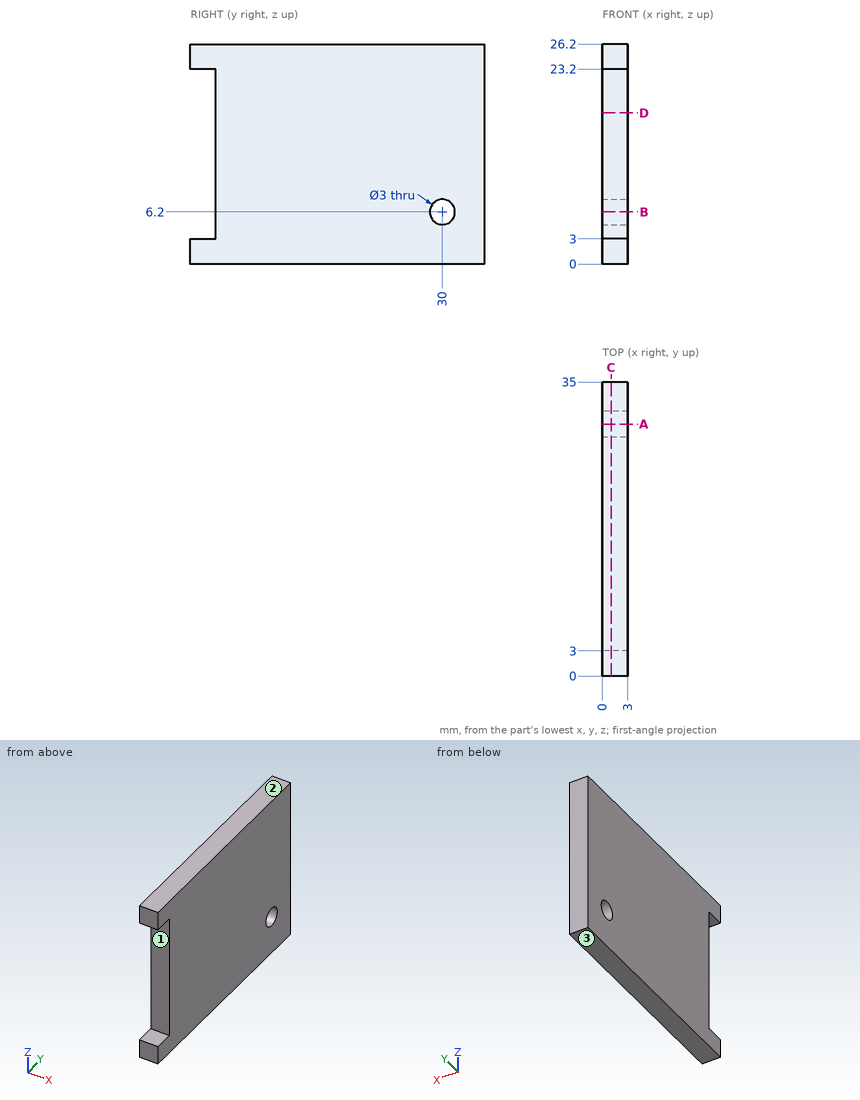
Can you work these out from the drawing? Everything is in mm from the part's minimum corner. Round coordinates to 2 decimals unless told otherwise and drop trailing zeros. Write each loop counter-clockwise with the first axis right and the second up, starting at its lowest first coordinate (ties: lowest second). Pieces come first, ordered by that corner, then holes. Notation, with made-up numbers: (28.25, -7.5) - (47.25, -7.5) arc R30 cw to (47.25, 19.5) - close; hole circle Ø9 at (-13.5, -17). An arc over 180 degrees is marked (long way). Put each result on its own line as item: value. Start each with the question number.
(1) I want a section at C-C, the plane x = 1.05. Please give me the cut outline in (y, z).
(2) I want a section at B-B, the plane z = 6.2. Please give me the cut outline in (x, y).
(3) Thinking about a two-plate mould opening in Z: for the marked faces 1, 2 and 3, which applies, released by +Z, released by -Z, zero draft, split by the parting line, or undercut?
(4) I need wall thicknesses on probe 1 along Z at (x, y) = (1.15, 30); probe 2 along Y at (x, z) = (0.5, 6.25); probe 3 along Y at (x, z) = (1.95, 8.25). Which ranges of each line are inside material? Lowest first, please.
(5) I want a section at A-A, the plane y = 30. Please give me the cut outline in (x, z), plus the area to 3 significant figures.
(6) I want a section at D-D, the plane z = 18. Please give me the cut outline in (x, y).
Here are the results:
1. outline: (0, 0) - (35, 0) - (35, 26.2) - (0, 26.2) - (0, 23.2) - (3, 23.2) - (3, 3) - (0, 3) - close; hole circle Ø3 at (30, 6.2)
2. outline: (0, 3) - (3, 3) - (3, 28.5) - (0, 28.5) - close; (0, 31.5) - (3, 31.5) - (3, 35) - (0, 35) - close
3. face 1: undercut
3. face 2: released by +Z
3. face 3: released by -Z
4. probe 1: z = 0 to 4.7, 7.7 to 26.2
4. probe 2: y = 3 to 28.5, 31.5 to 35
4. probe 3: y = 3 to 35
5. outline: (0, 0) - (3, 0) - (3, 4.7) - (0, 4.7) - close; (0, 7.7) - (3, 7.7) - (3, 26.2) - (0, 26.2) - close
5. area: 69.6 mm^2
6. outline: (0, 3) - (3, 3) - (3, 35) - (0, 35) - close
